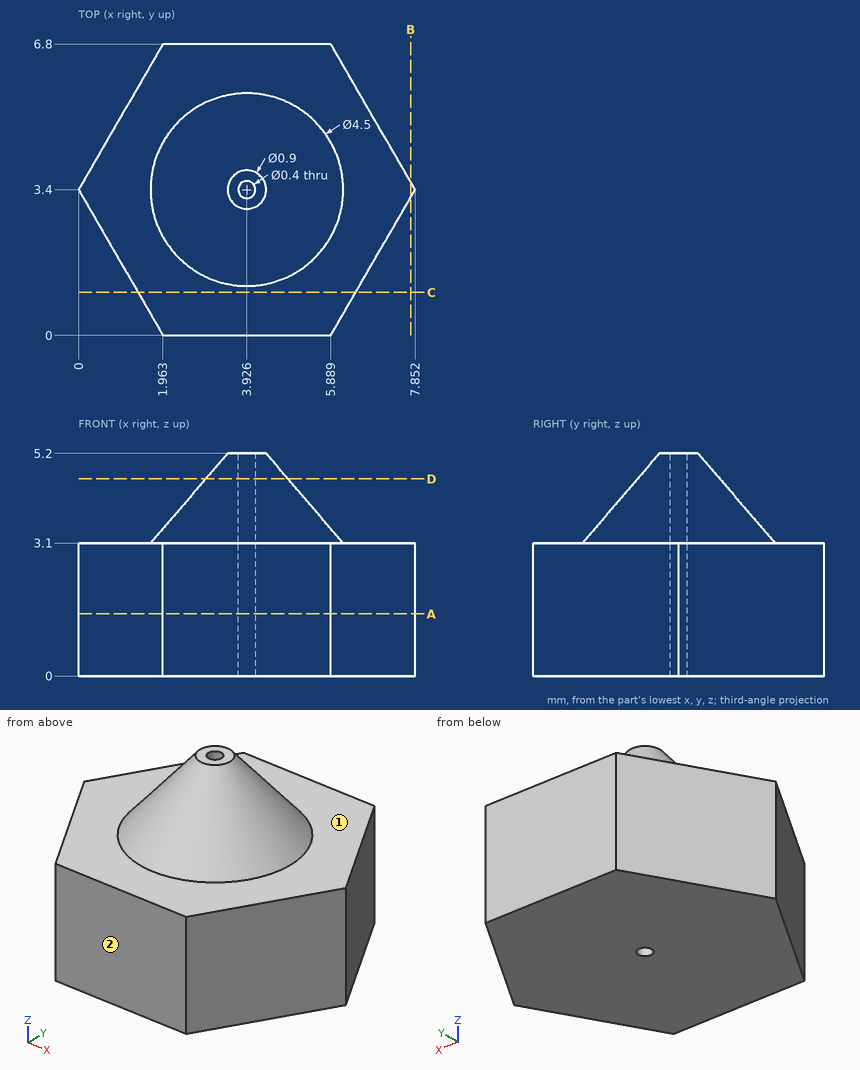
The figure shows three views and two pictorial views of one solid part (mm, origin at its lowest corner). Answer the questions. A direction names the side the tool comes from. Give positions to 0.01 mm unless a question says otherwise; leave off trailing zeros. Order: outer loops, then holes, each group sorted by start corner. A loop starts at its lowest first (then second) coordinate and runs counter-clockwise, first axis right, second up. Notation, with made-up numbers: (1.5, -6) - (11.5, -6) arc R23 ccw to (11.5, 11) - close; hole circle Ø6 at (40, -27). An arc over 180 degrees is marked (long way). Answer as CSV lines item,"result".
Q1. A cutting plane is placed at B-B, the plane x = 7.75. Determine the outline of the cut face in (y, z).
Answer key:
outline,"(3.22, 0) - (3.58, 0) - (3.58, 3.1) - (3.22, 3.1) - close"
Q2. Which of the six approach directions +Z, -Z, +X, -X, +Y, -Y give full straight-line access (tool end or side, diameter ignored) to the marked faces 1 and 2?
Answer key:
face 1,"+Z"
face 2,"+Z, -Z, +X, -X, -Y"
Q3. A cutting plane is placed at A-A, the plane z = 1.45. Determine the outline of the cut face in (x, y), and give its area (3 significant figures).
Answer key:
outline,"(0, 3.4) - (1.96, 0) - (5.89, 0) - (7.85, 3.4) - (5.89, 6.8) - (1.96, 6.8) - close; hole circle Ø0.4 at (3.93, 3.4)"
area,"39.9 mm^2"
Q4. A cutting plane is placed at D-D, the plane z = 4.6. Determine the outline of the cut face in (x, y).
Answer key:
outline,"circle Ø1.93 at (3.93, 3.4); hole circle Ø0.4 at (3.93, 3.4)"
Q5. A cutting plane is placed at C-C, the plane y = 1. Determine the outline of the cut face in (x, z).
Answer key:
outline,"(1.39, 0) - (6.47, 0) - (6.47, 3.1) - (1.39, 3.1) - close"
Q6. Each of these flat-tipped pins is pushed along its axis until it touches: pin 1 Ø1 at (y, z) = (5.5, 2.5) entering from +X; pin 2 Ø1 at (y, z) = (2, 3) entering from -X. Where does it stop, or does it pass through?
Answer key:
pin 1,"stops at x = 6.93"
pin 2,"stops at x = 0.52"
Q7. Straight lines are drawn through the part: L1, parallel to Z at x = 6.75, y = 3.75; L2, parallel to Y at x = 4, z = 3.6; L3, parallel to X at y = 0.5, z = 2.35. For each, find the intervals that lie inside material, in ascending order.
Answer key:
L1,"z = 0 to 3.1"
L2,"y = 1.58 to 3.21, 3.59 to 5.22"
L3,"x = 1.67 to 6.18"
